Study the drawing (mm; zero at the part's minimum x, y, z) and answer. A direction names the side the tool comes from. Coordinates: 2 decimals unless noted, no trailing zeros. Order: outer loops, then holes, each group sorted by start corner. A loop starts at its lowest first (then second) coordinate and runs counter-clockwise, first axis right, second up. Notation, with made-up numbers: (23.25, 6) -> (46.25, 6) arc R23 ccw to (46.25, 14) -> close; hole circle Ø3 at (-15, 60.25). An arc over 180 degrees is marked (long way). Answer in a Markdown table with one row per item. Add a question column.
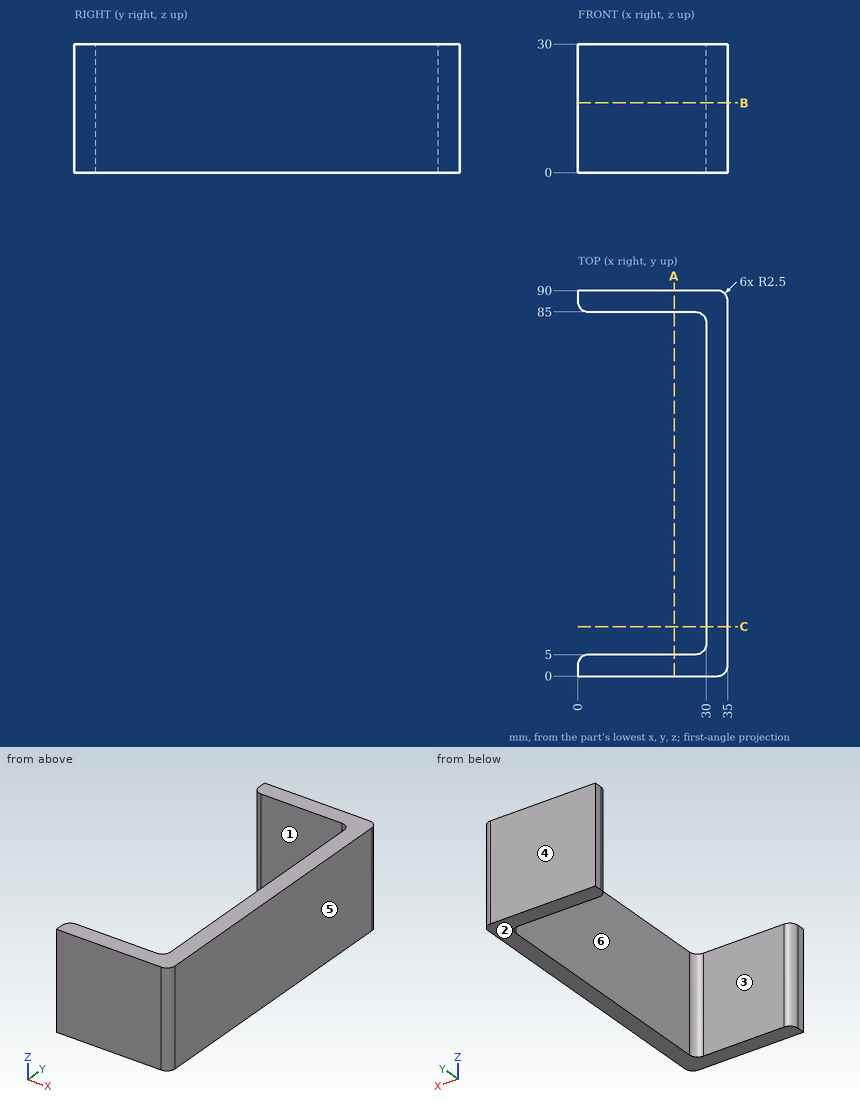
Q1. Straight lines are drawn through the part: line 1 (Y direction, x = 26.5, z = 11.25); line 2 (X direction, y = 54.5, z = 7.5); line 3 (Y direction, x = 29.5, z = 22). For each, find the intervals that lie inside material, in ascending order.
Q2. Determine the mould class of the marked faces 3, 4, 5 and 6 for opening direction Y: +Y half, -Y half, draft (parallel to the pull), parting line (faces both ways), or undercut.
Q3. A cutting plane is placed at B-B (z = 16.25). Determine the outline of the cut face in (x, y).
Q4. A cutting plane is placed at C-C (y = 11.5). Determine the outline of the cut face in (x, z).
Q5. For the marked faces 1 and 2, determine the directions among +Z, -Z, +X, -X, +Y, -Y from which every point of the face is accessible in a straight line to the end or side of a thin tool.
Q6. A cutting plane is placed at A-A (x = 22.5). Determine the outline of the cut face in (y, z), then the cut area to 3 significant figures.
Q7. Given pin 1 (8 mm diameter, centred on y = 73, z = 17.5, fed in from -X), flat-ended and moving along its own axis, determine where the tip first touches the part or whether it passes through.
Returned:
| question | item | result |
|---|---|---|
| 1 | line 1 | y = 0 to 5, 85 to 90 |
| 1 | line 2 | x = 30 to 35 |
| 1 | line 3 | y = 0 to 6, 84 to 90 |
| 2 | face 3 | undercut |
| 2 | face 4 | +Y half |
| 2 | face 5 | draft |
| 2 | face 6 | undercut |
| 3 | outline | (0, 0) -> (32.5, 0) arc R2.5 ccw to (35, 2.5) -> (35, 87.5) arc R2.5 ccw to (32.5, 90) -> (0, 90) -> (0, 87.5) arc R2.5 ccw to (2.5, 85) -> (27.5, 85) arc R2.5 cw to (30, 82.5) -> (30, 7.5) arc R2.5 cw to (27.5, 5) -> (2.5, 5) arc R2.5 ccw to (0, 2.5) -> close |
| 4 | outline | (30, 0) -> (35, 0) -> (35, 30) -> (30, 30) -> close |
| 5 | face 1 | +Z, -Z, -X |
| 5 | face 2 | -Z, +X, -X, +Y, -Y |
| 6 | outline | (0, 0) -> (5, 0) -> (5, 30) -> (0, 30) -> close; (85, 0) -> (90, 0) -> (90, 30) -> (85, 30) -> close |
| 6 | area | 300 mm² |
| 7 | pin 1 | stops at x = 30 |
